Work out the finished part from the listing and answer in its coordinate system (mm). Face numbers are marked on the shaded views. A direction names the side the tool comes from. Round coordinates to 2 decimals unless told otherwise and drop trailing zeros. Loops run counter-clockwise (first coordinate to the right, second up) from the corner with the lowest first, then second, coordinate; pieces in that order, holes last. Notation, with made-up numbers: (-13, 84) - (7, 84) arc R28 ccw to (7, 103) - close; hole circle Ø4 at (20.25, 77.5). An arc over 180 degrees is marked (long way). Answer as CSV lines item,"result". Start each with the question number.
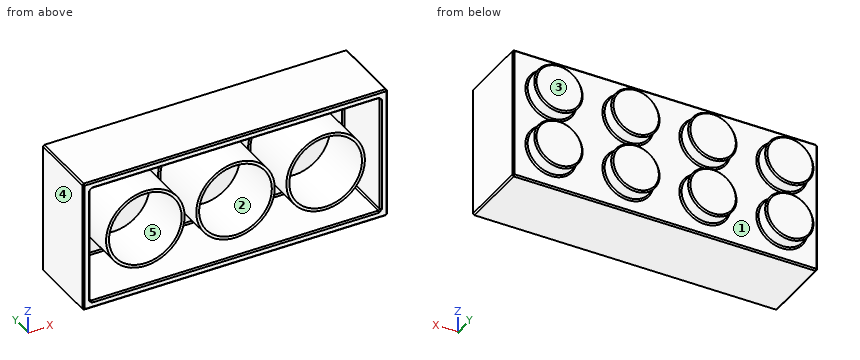
```python
from build123d import *

# Parameters (mm, degrees)
SKETCH_W        = 199.522308
SKETCH_H        = 80.891732
PAD_DEPTH       = 45
THICKNESS_T     = 5
SKETCH001_R     = 27
PAD001_DEPTH    = 45
SKETCH002_R     = 25
POCKET_DEPTH    = 40
CHAMFER_SIZE    = 1
CHAMFER001_SIZE = 1
SKETCH003_R     = 16.619599
PAD002_DEPTH    = 10
CHAMFER002_SIZE = 1
CHAMFER003_SIZE = 1


with BuildPart() as part:
    # Sketch → Pad (new body)
    with BuildSketch(Plane.XZ):
        Rectangle(SKETCH_W, SKETCH_H)
    extrude(amount=PAD_DEPTH)

    # Thickness
    thickness_openings = [part.faces().sort_by_distance(p)[0] for p in [
        (0, -45, 0),
    ]]
    offset(amount=THICKNESS_T, openings=thickness_openings, kind=Kind.INTERSECTION)

    # Sketch001 (on Face5 of Thickness) → Pad001 (join)
    with BuildSketch(Plane.XZ):
        Circle(SKETCH001_R)
        with Locations((62, 0)):
            Circle(SKETCH001_R)
        with Locations((-62, 0)):
            Circle(SKETCH001_R)
    extrude(amount=PAD001_DEPTH)

    # Sketch002 → Pocket (cut)
    with BuildSketch(Plane.XZ.offset(46)):
        Circle(SKETCH002_R)
        with Locations((-62, 0)):
            Circle(SKETCH002_R)
        with Locations((62, 0)):
            Circle(SKETCH002_R)
    extrude(amount=-POCKET_DEPTH, mode=Mode.SUBTRACT)

    # Chamfer
    chamfer_edges = [part.edges().sort_by_distance(p)[0] for p in [
        (-99.761154, 0, 0),
        (0, 0, -40.445866),
        (0, 0, 40.445866),
        (99.761154, 0, 0),
        (-89, 0, 0),
        (-27, 0, 0),
        (35, 0, 0),
        (-99.761154, -22.5, 40.445866),
        (99.761154, -22.5, 40.445866),
        (0, -45, 40.445866),
        (-99.761154, -22.5, -40.445866),
        (-99.761154, -45, 0),
        (99.761154, -22.5, -40.445866),
        (99.761154, -45, 0),
        (0, -45, -40.445866),
    ]]
    chamfer(chamfer_edges, length=CHAMFER_SIZE)

    # Chamfer001
    chamfer001_edges = [part.edges().sort_by_distance(p)[0] for p in [
        (104.761154, -20, 45.445866),
        (0, 5, 45.445866),
        (-104.761154, -20, 45.445866),
        (0, -45, 45.445866),
        (104.761154, -20, -45.445866),
        (104.761154, 5, 0),
        (104.761154, -45, 0),
        (-104.761154, 5, 0),
        (0, 5, -45.445866),
        (-104.761154, -20, -45.445866),
        (-104.761154, -45, 0),
        (0, -45, -45.445866),
    ]]
    chamfer(chamfer001_edges, length=CHAMFER001_SIZE)

    # Sketch003 (on Face48 of Chamfer001) → Pad002 (join)
    with BuildSketch(Plane(origin=(0, 5, 0), x_dir=(-1, 0, 0), z_dir=(0, 1, 0))):
        with Locations((-78.721924, 20.108581)):
            Circle(SKETCH003_R)
        with Locations((-25.795449, 20.108581)):
            Circle(SKETCH003_R)
        with Locations((27.131026, 20.108581)):
            Circle(SKETCH003_R)
        with Locations((80.0575, 20.108581)):
            Circle(SKETCH003_R)
        with Locations((-78.721924, -19.88926)):
            Circle(SKETCH003_R)
        with Locations((-25.795449, -19.88926)):
            Circle(SKETCH003_R)
        with Locations((27.131026, -19.88926)):
            Circle(SKETCH003_R)
        with Locations((80.0575, -19.88926)):
            Circle(SKETCH003_R)
    extrude(amount=PAD002_DEPTH)

    # Chamfer002
    chamfer002_edges = [part.edges().sort_by_distance(p)[0] for p in [
        (-63.437902, 15, 20.108581),
        (-63.437902, 15, -19.88926),
        (-10.511427, 15, -19.88926),
        (-10.511427, 15, 20.108581),
        (42.415048, 15, 20.108581),
        (42.415048, 15, -19.88926),
        (95.341523, 15, -19.88926),
        (95.341523, 15, 20.108581),
    ]]
    chamfer(chamfer002_edges, length=CHAMFER002_SIZE)

    # Chamfer003
    chamfer003_edges = [part.edges().sort_by_distance(p)[0] for p in [
        (-10.511427, 5, 20.108581),
        (-10.511427, 5, -19.88926),
        (42.415048, 5, -19.88926),
        (42.415048, 5, 20.108581),
        (95.341523, 5, -19.88926),
        (95.341523, 5, 20.108581),
        (-63.437902, 5, -19.88926),
        (-63.437902, 5, 20.108581),
    ]]
    chamfer(chamfer003_edges, length=CHAMFER003_SIZE)


solid = part.part
```
Item 1: Determine the mould class of the marked faces 4 and 5 for opening direction Z: pulls with the +Z half, pulls with the -Z half, needs draft (parallel to the pull), parting line crosses it, or undercut.
Item 2: Find the intervals of material crossed by L1, parallel to Z at x = 62, y = -21; L2, parallel to X at y = -39.5, z = -32; L3, parallel to Z at x = -73, y = -8.5, in increasing order.
Item 3: Section B-B, the plane x = 0 is taken. Give the vertices of the cut face in (y, z).
Item 4: Section A-A, the plane y = -34.5 is taken. Give the vertices of the cut face in (x, z), and give its area (3 significant figures).
Item 5: Which of the six approach directions +Z, -Z, +X, -X, +Y, -Y give full straight-line access (tool end or side, diameter ignored) to the marked faces 1, 2 and 3?
Answer:
1,face 4,"needs draft"
1,face 5,"undercut"
2,L1,"z = -45.45 to -40.45, -27 to -25, 25 to 27, 40.45 to 45.45"
2,L2,"x = -104.76 to -99.76, 99.76 to 104.76"
2,L3,"z = -45.45 to -40.45, -24.66 to -22.45, 22.45 to 24.66, 40.45 to 45.45"
3,outline,"(-45, -44.45) - (-44, -45.45) - (4, -45.45) - (5, -44.45) - (5, 44.45) - (4, 45.45) - (-44, 45.45) - (-45, 44.45) - (-45, 41.45) - (-44, 40.45) - (-1, 40.45) - (0, 39.45) - (0, 28) - (-1, 27) - (-45, 27) - (-45, 25) - (-6, 25) - (-6, -25) - (-45, -25) - (-45, -27) - (-1, -27) - (0, -28) - (0, -39.45) - (-1, -40.45) - (-44, -40.45) - (-45, -41.45) - close"
4,outline,"(-104.76, -44.45) - (-103.76, -45.45) - (103.76, -45.45) - (104.76, -44.45) - (104.76, 44.45) - (103.76, 45.45) - (-103.76, 45.45) - (-104.76, 44.45) - close; circle Ø54 at (-62, 0); circle Ø54 at (0, 0); circle Ø54 at (62, 0); hole (-99.76, -39.45) - (-98.76, -40.45) - (98.76, -40.45) - (99.76, -39.45) - (99.76, 39.45) - (98.76, 40.45) - (-98.76, 40.45) - (-99.76, 39.45) - close; hole circle Ø50 at (-62, 0); hole circle Ø50 at (0, 0); hole circle Ø50 at (62, 0)"
4,area,"3,880 mm²"
5,face 1,"+Y"
5,face 2,"-Y"
5,face 3,"+Z, -Z, +X, -X, +Y"
